Could you check a few things on this drawing? It's one solid part, dimensions in mm from its lowest x, y, z. A direction names the side the tool comes from. Give positions to 0.01 mm unless a question says otherwise; leave off trailing zeros. Loops run counter-clockwise (first coordinate to the right, second up) from the corner with the lowest first, then second, coordinate; pieces in that order, holes last. Notation, with made-up numbers: (47, 75.25) -> (78, 75.25) arc R12 cw to (78, 87.25) -> close; hole circle Ø8 at (59.25, -27.5). An arc over 180 degrees is marked (long way). One line per question, with ' | ' between items.
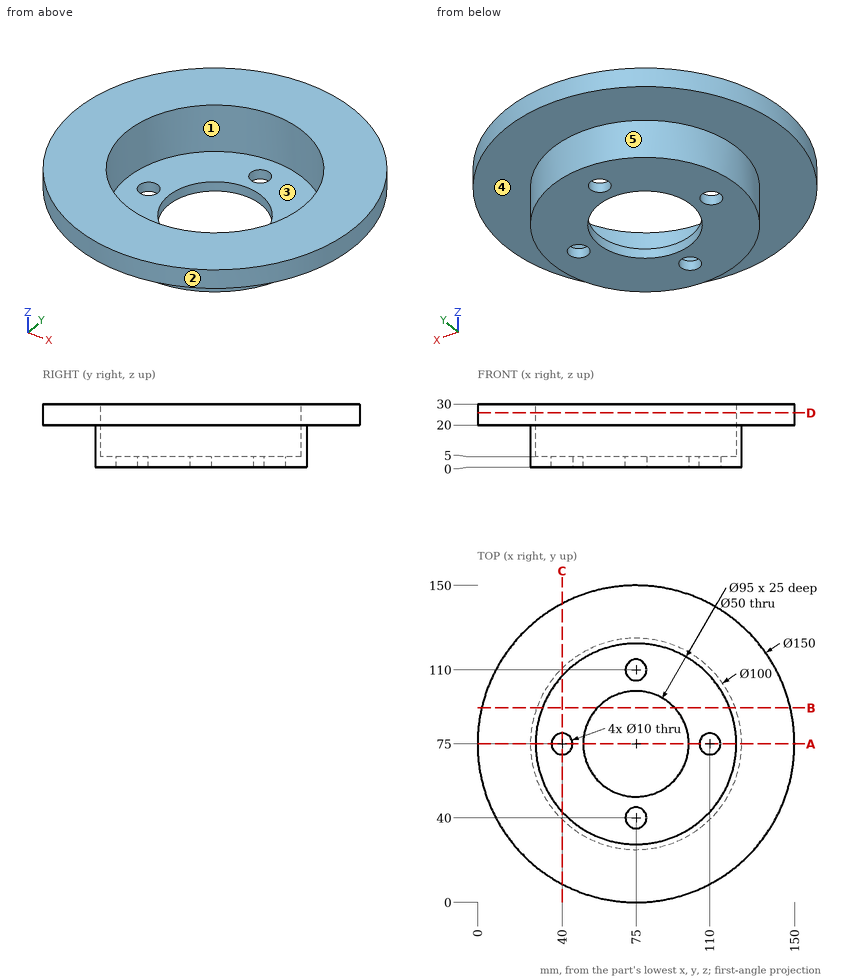
Q1. If we section it at D-D (z = 25.75): Write out the boundary of the cut face in (x, y), plus the area to 3 significant figures.
Entries:
outline: circle Ø150 at (75, 75); hole circle Ø95 at (75, 75) | area: 10,600 mm²
Q2. On a 3-axis mill with a long thin cutter (end or side, diameter ignored), from which of +Z, -Z, +X, -X, +Y, -Y can I reach the whole of each face in a straight line? I mean the marked faces 1 and 2. Say none if no direction works.
Entries:
face 1: +Z | face 2: +Z, -Z
Q3. If we mould it in two halves opening along Y, with no side actions, what happens to the marked faces 3, 4 and 5? For each: pulls with the +Y half, pulls with the -Y half, needs draft (parallel to the pull), parting line crosses it, or undercut.
Entries:
face 3: undercut | face 4: needs draft | face 5: parting line crosses it
Q4. If we section it at A-A (y = 75): Write out the boundary of the cut face in (x, z).
Entries:
outline: (0, 20) -> (25, 20) -> (25, 0) -> (35, 0) -> (35, 5) -> (27.5, 5) -> (27.5, 30) -> (0, 30) -> close; (45, 0) -> (50, 0) -> (50, 5) -> (45, 5) -> close; (100, 0) -> (105, 0) -> (105, 5) -> (100, 5) -> close; (115, 0) -> (125, 0) -> (125, 20) -> (150, 20) -> (150, 30) -> (122.5, 30) -> (122.5, 5) -> (115, 5) -> close
Q5. If we section it at C-C (x = 40): Write out the boundary of the cut face in (y, z).
Entries:
outline: (8.67, 20) -> (39.29, 20) -> (39.29, 0) -> (70, 0) -> (70, 5) -> (42.89, 5) -> (42.89, 30) -> (8.67, 30) -> close; (80, 0) -> (110.71, 0) -> (110.71, 20) -> (141.33, 20) -> (141.33, 30) -> (107.11, 30) -> (107.11, 5) -> (80, 5) -> close
Q6. If I drill on probe 1 along Z at (x, y) = (24, 59); probe 2 along Y at (x, z) = (63.5, 27.75); probe 3 along Y at (x, z) = (104, 14.75), over which ranges is the centre line in solid material (lowest first)? Write a range as from..to.
Entries:
probe 1: 20..30 | probe 2: 0.89..28.91, 121.09..149.11 | probe 3: 34.27..37.38, 112.62..115.73
Q7. If we section it at B-B (y = 92): Write out the boundary of the cut face in (x, z).
Entries:
outline: (1.95, 20) -> (27.98, 20) -> (27.98, 0) -> (56.67, 0) -> (56.67, 5) -> (30.65, 5) -> (30.65, 30) -> (1.95, 30) -> close; (93.33, 0) -> (122.02, 0) -> (122.02, 20) -> (148.05, 20) -> (148.05, 30) -> (119.35, 30) -> (119.35, 5) -> (93.33, 5) -> close
Q8. For pin 1 Ø1 at (y, z) = (33, 14.5) entering from +X; pin 2 Ø1 at (x, z) = (69, 12.5) entering from -Y; pin 3 Ø5 at (x, z) = (37.5, 11) entering from -Y, each with a flat end and sliding along its axis, tell me the tip position at first contact or that it passes through.
Entries:
pin 1: x = 102.89 | pin 2: y = 25.3 | pin 3: y = 39.29
